Design review of the part shown in the three views and the two pictorial views. Dimensions are in mm from the part's minimum x, y and z. A direction names the side the tool comes from. Give positions to 0.01 mm unless a question says otherwise; leave off trailing zeros. Write each loop counter-clockwise with the first axis right and the second up, starting at its lowest first coordinate (ties: lowest second). Pieces come first, ordered by that corner, then holes.
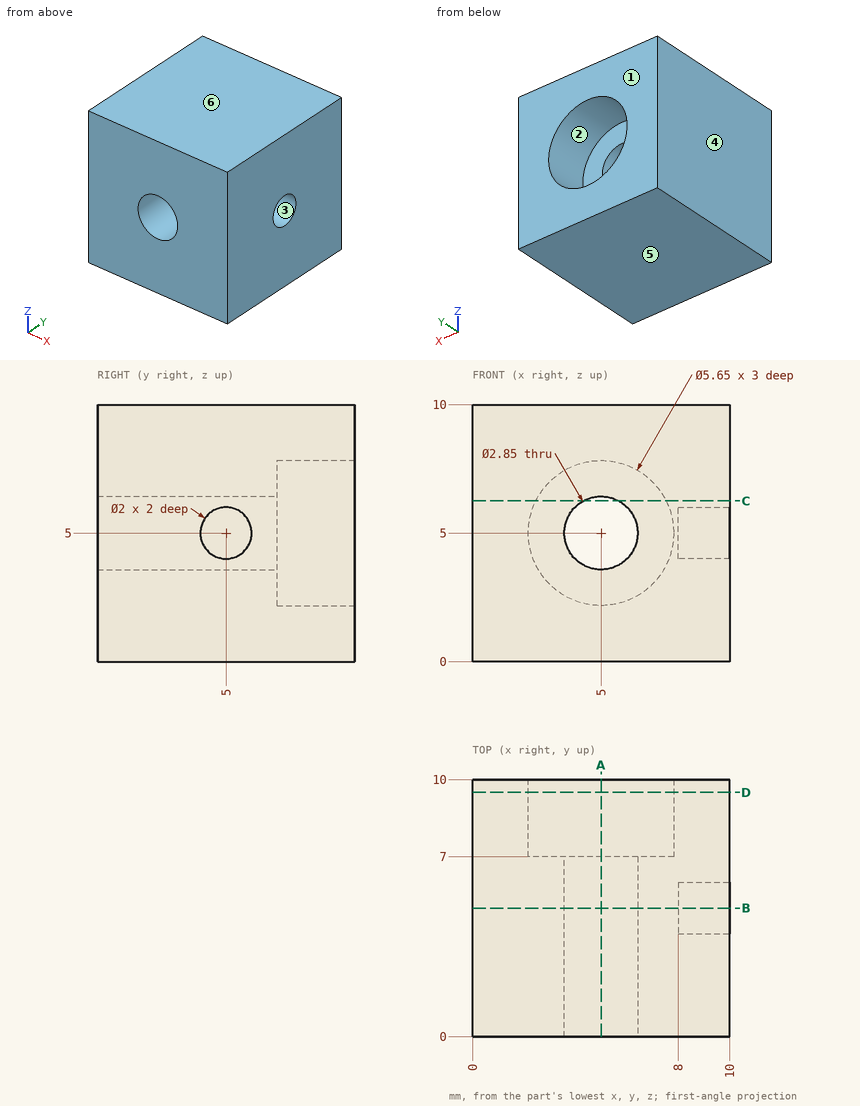
(1) Consider section D-D, the plane y = 9.5. Give the boundary of the cut face in (x, z) (3 decimals).
Resolved:
outline: (0, 0) - (10, 0) - (10, 10) - (0, 10) - close; hole circle Ø5.65 at (5, 5)
(2) Consider section B-B, the plane y = 5. Give the boundary of the cut face in (x, z) (3 decimals), then the cut area to 3 significant figures.
Resolved:
outline: (0, 0) - (10, 0) - (10, 4) - (8, 4) - (8, 6) - (10, 6) - (10, 10) - (0, 10) - close; hole circle Ø2.85 at (5, 5)
area: 89.6 mm2
(3) Clearance check with flat-ended pins moving along their axes: P1, Ø4, axis at x = 4.5, z = 5, coming from the +Y side; P2, Ø1.8, axis at y = 5, z = 5, coming from the +X side. State where each tip first meets the part, or that it passes through.
Resolved:
P1: stops at y = 7
P2: stops at x = 8
(4) To check wall thickness, follow L1, parallel to X at y = 3.75, z = 5 (3 decimals); L2, parallel to Y at x = 9.4, z = 5; L3, parallel to X at y = 4.75, z = 5 (3 decimals). State the ranges of each line that lie inside material, in increasing order.
Resolved:
L1: x = 0 to 3.575, 6.425 to 10
L2: y = 0 to 4, 6 to 10
L3: x = 0 to 3.575, 6.425 to 8
(5) Tool access review of the marked faces 1 and 2: name each direction out of +Z, -Z, +X, -X, +Y, -Y from which nothing blocks a thin tool from reaching the whole face with its end or side.
Resolved:
face 1: +Z, -Z, +X, -X, +Y
face 2: +Y
(6) Consider section A-A, the plane x = 5. Give the boundary of the cut face in (y, z) (3 decimals).
Resolved:
outline: (0, 0) - (10, 0) - (10, 2.175) - (7, 2.175) - (7, 3.575) - (0, 3.575) - close; (0, 6.425) - (7, 6.425) - (7, 7.825) - (10, 7.825) - (10, 10) - (0, 10) - close
(7) Consider section C-C, the plane z = 6.25. Give the boundary of the cut face in (x, y), then the cut area to 3 significant figures.
Resolved:
outline: (0, 0) - (4.32, 0) - (4.32, 7) - (2.47, 7) - (2.47, 10) - (0, 10) - close; (5.68, 0) - (10, 0) - (10, 10) - (7.53, 10) - (7.53, 7) - (5.68, 7) - close
area: 75.2 mm2
(8) Mouldability with a two-part tool opening along Z and no side actions: class the marked faces 3, 4, 5 and 6 as pulls with the +Z half, pulls with the -Z half, needs draft (parallel to the pull), parting line crosses it, or undercut.
Resolved:
face 3: undercut
face 4: needs draft
face 5: pulls with the -Z half
face 6: pulls with the +Z half
